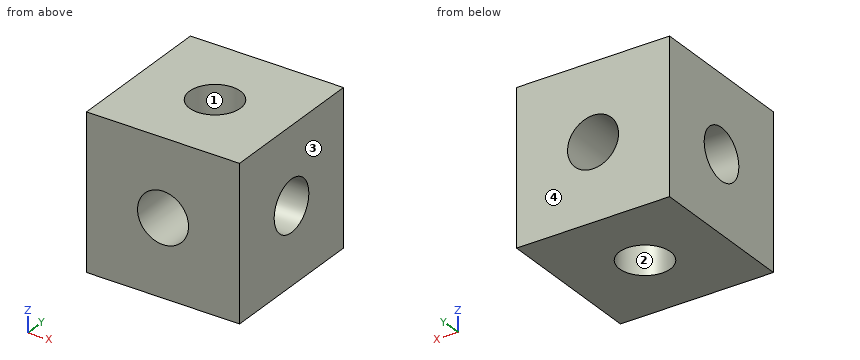
from build123d import *

# Parameters (mm, degrees)
SKETCH1_W           = 15
SKETCH1_H           = 15
BOSS_EXTRUDE1_DEPTH = 15
SKETCH3_R           = 2.5
CUT_EXTRUDE1_DEPTH  = 19.371173071
SKETCH4_R           = 2.5
CUT_EXTRUDE2_DEPTH  = 23.5
SKETCH5_R           = 2.5
CUT_EXTRUDE3_DEPTH  = 23.5


with BuildPart() as part:
    # Sketch1 → Boss-Extrude1 (new body)
    with BuildSketch(Plane(origin=(0, 0, 0), x_dir=(1, 0, 0), z_dir=(0, 1, 0))):
        Rectangle(SKETCH1_W, SKETCH1_H)
    extrude(amount=BOSS_EXTRUDE1_DEPTH)

    # Sketch3 → Cut-Extrude1 (cut, through all)
    with BuildSketch(Plane(origin=(0, 15, 0), x_dir=(1, 0, 0), z_dir=(0, 1, 0))):
        with Locations(Location((0, 0, 0), (0, 0, 270))):
            Circle(SKETCH3_R)
    extrude(amount=-CUT_EXTRUDE1_DEPTH, mode=Mode.SUBTRACT)

    # Sketch4 → Cut-Extrude2 (cut, through all)
    with BuildSketch(Plane.ZY.offset(7.5)):
        with Locations((0, 7.5)):
            Circle(SKETCH4_R)
    extrude(amount=-CUT_EXTRUDE2_DEPTH, mode=Mode.SUBTRACT)

    # Sketch5 → Cut-Extrude3 (cut, through all)
    with BuildSketch(Plane.XY.offset(7.5)):
        with Locations((0, 7.5)):
            Circle(SKETCH5_R)
    extrude(amount=-CUT_EXTRUDE3_DEPTH, mode=Mode.SUBTRACT)


solid = part.part
Work out the finished part from the listing and answer in its coordinate system (mm). Face numbers are marked on the shaded views. Coordinates: 2 decimals unless noted, no trailing zeros. Write each loop counter-clockwise with the first axis right and the second up, starting at its lowest first coordinate (ties: lowest second). Pieces come first, ordered by that corner, then holes. Notation, with made-up numbers: M 43.5,80 L 79.5,80 A14 ccw 79.5,102 Z; hole C -12.75,61.5 d1. An arc over 180 degrees is marked long. Write item = value, one per line.
1. The part is cut by section D-D (x = 5). Determine the outline of the cut face in (y, z).
Solution:
outline = M 0,-7.5 L 15,-7.5 L 15,7.5 L 0,7.5 Z; hole C 7.5,0 d5
2. The part is cut by section C-C (z = -5.5). Determine the outline of the cut face in (x, y), then the cut area to 3 significant figures.
Solution:
outline = M -7.5,0 L 7.5,0 L 7.5,15 L -7.5,15 Z; hole C 0,7.5 d5
area = 205 mm2
3. The part is cut by section B-B (y = 7.5). Determine the outline of the cut face in (x, z), then the cut area to 3 significant figures.
Solution:
outline = M -7.5,-7.5 L -2.5,-7.5 L -2.5,-2.5 L -7.5,-2.5 Z; M -7.5,2.5 L -2.5,2.5 L -2.5,7.5 L -7.5,7.5 Z; M 2.5,-7.5 L 7.5,-7.5 L 7.5,-2.5 L 2.5,-2.5 Z; M 2.5,2.5 L 7.5,2.5 L 7.5,7.5 L 2.5,7.5 Z
area = 100 mm2
4. Determine the mould class of the marked faces 1, 2, 3 and 4 for opening direction X: released by +X, released by -X, zero draft, split by the parting line, or undercut.
Solution:
face_1 = undercut
face_2 = undercut
face_3 = released by +X
face_4 = zero draft
5. Straight lines are drawn through the part: line 1 (Y direction, x = 0, z = 5.15); line 2 (Z direction, x = -3, y = 7.5); line 3 (Y direction, x = -0.75, z = 3.25). For each, find the intervals that lie inside material, in ascending order. Write a range as from..to.
Solution:
line_1 = 0..5, 10..15
line_2 = -7.5..-2.5, 2.5..7.5
line_3 = 0..5.12, 9.88..15
6. The part is cut by section A-A (z = 0). Determine the outline of the cut face in (x, y), then the cut area to 3 significant figures.
Solution:
outline = M -7.5,0 L -2.5,0 L -2.5,5 L -7.5,5 Z; M -7.5,10 L -2.5,10 L -2.5,15 L -7.5,15 Z; M 2.5,0 L 7.5,0 L 7.5,5 L 2.5,5 Z; M 2.5,10 L 7.5,10 L 7.5,15 L 2.5,15 Z
area = 100 mm2
